Design review of the part shown in the three views and the two pictorial views. Dimensions are in mm from the part's minimum x, y and z. Coordinates: 2 decimals unless noted, no trailing zeros. Write each loop counter-clockwise with the first axis right and the second up, starting at its lowest first coordinate (ties: lowest second). Pieces come first, ordered by that corner, then holes. Notation, with made-up numbers: (11, -7) -> (54, -7) arc R20 cw to (54, 21) -> close; hole circle Ø7 at (19, 30). An arc over 180 degrees is marked (long way). Answer in a Markdown table with one row per item. Add a question column.
Item 1: Clearance check with a flat-ended pin moving along its axis: P1, Ø1.5, axis at x = 35, y = 38.5, coming from the -Z side. State where the tip first meets the part, or that it passes through.
Item 2: To check wall thickness, follow line 1 (Y direction, x = 31, z = 0.1); line 2 (Y direction, x = 29, z = 1.4). State the ranges of each line that lie inside material, in increasing order.
Item 3: Take a section at A-A, the plane x = 29. Write out the cut boundary in (y, z), and give its area (3 significant figures).
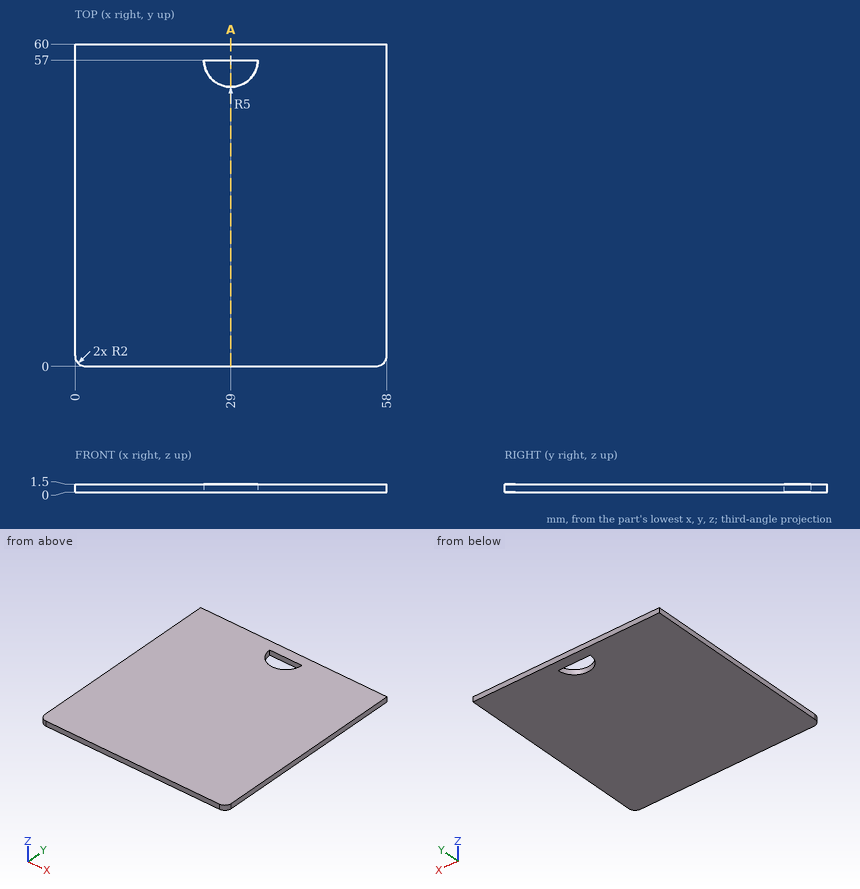
Answers:
| question | item | result |
|---|---|---|
| 1 | P1 | stops at z = 0 |
| 2 | line 1 | y = 0 to 52.42, 57 to 60 |
| 2 | line 2 | y = 0 to 52, 57 to 60 |
| 3 | outline | (0, 0) -> (52, 0) -> (52, 1.5) -> (0, 1.5) -> close; (57, 0) -> (60, 0) -> (60, 1.5) -> (57, 1.5) -> close |
| 3 | area | 82.5 mm^2 |
